The model under review builds one solid part; all positions refer to its coordinate system, in mm. Face numbers are marked on the shaded views. A direction names the side the tool comes from. Round coordinates to 2 decimals unless told otherwise and drop trailing zeros. Loops run counter-clockwise (first coordinate to the right, second up) from the corner with the lowest first, then second, coordinate; pieces in that order, holes last. Notation, with made-up numbers: M 34.25,-39.75 L 90.25,-39.75 A35 ccw 90.25,-1.75 Z; hole C 54,-19 d5. An arc over 180 degrees is marked long. Return JSON: item names as keys, results as strings. Group by question number.
Q1. Consider section B-B (z = 17). State the section outline as (x, y) points.
Q2. Clearance check with flat-ended pins moving along their axes: pin 1 Ø12.5 at (x, y) = (32, -1.5) entering from -Z; pin 2 Ø2 at (y, z) = (-8.5, 25.5) entering from +X; pin 3 Ø1.5 at (x, z) = (-12.5, 25) entering from +Y; pin 4 Ø2 at (x, z) = (13.5, 22.5) entering from -Y. State where each tip first meets the part, or that it passes through.
Q3. Consider section A-A (y = 24). State the section outline as (x, z) points, and give its area (3 significant figures).
Q4. Consider section D-D (y = -18). State the section outline as (x, z) points.
Q5. Consider section C-C (x = 38.5). State the section outline as (y, z) points.
Q6. To check wall thickness, follow line 1 along X through (y, z) = (17, 23.5); line 2 along Z through (x, y) = (73, 24); line 3 along Z through (x, y) = (-33.5, 21.5). State the ranges of each line that lie inside material, in increasing order.
Q7. For the marked faces 1 and 2, list the 3-axis set-ups (+Z, -Z, +X, -X, +Y, -Y) from which the entire face can be reached by the end or side of a thin tool; tool diameter is ignored.
from build123d import *

# Parameters (mm, degrees)
F1_DEPTH = 72
F3_DEPTH = 2
F4_W     = 23
F4_H     = 4
F5_DEPTH = 25


# Not quite as in the source:
# - a pattern or mirror of a feature is missing from the dataset's text; its kind, count and spacing are read off the source's solid


with BuildPart() as f1:
    # F0 (on Right) → F1 (new body, symmetric)
    with BuildSketch(Plane.YZ):
        Polygon((-22, 23), (-20, 23), (-20, 25), (20, 25), (20, 21), (22, 21), (22, 27), (-22, 27), align=None)
    extrude(amount=F1_DEPTH, both=True)

    # F2 (on face) → F3 (join)
    with BuildSketch(Plane.YZ.offset(72)):
        with BuildLine():
            Line((30, 27), (22, 27))
            Line((22, 27), (8, 27))
            ThreePointArc((8, 27), (12.2327735284, 20.5611792354), (13.7171431429, 13))
            Line((13.7171431429, 13), (22, 13))
            Line((22, 13), (22, 14.7639320225))
            ThreePointArc((22, 14.7639320225), (24, 20), (26, 14.7639320225))
            Line((26, 14.7639320225), (26, 13))
            Line((26, 13), (30, 13))
            Line((30, 13), (30, 27))
        make_face()
    f3 = extrude(amount=F3_DEPTH)

    # F3_copies: F3 across plane
    add(f3.mirror(Plane(origin=(0, 0, 0), x_dir=(0, 0, -1), z_dir=(-1, 0, 0))))

    # F4 (on face) → F5 (cut)
    with BuildSketch(Plane(origin=(0, 22, 0), x_dir=(-1, 0, 0), z_dir=(0, 1, 0))):
        with Locations((46.5, 23)):
            Rectangle(F4_W, F4_H)
    extrude(amount=-F5_DEPTH, mode=Mode.SUBTRACT)


solid = f1.part
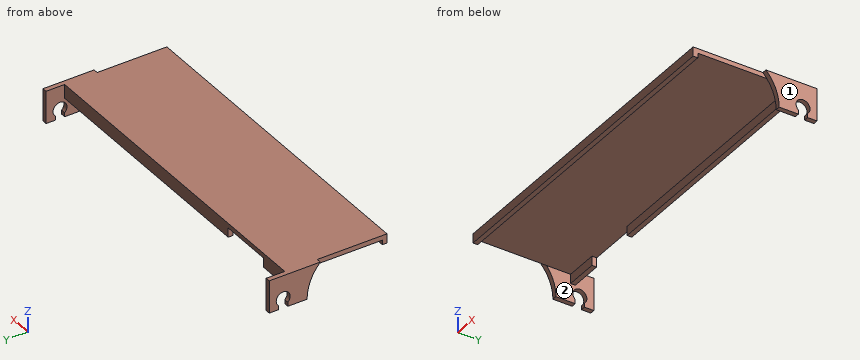
Values:
{
 "1": {"outline": "M -74,13.31 L -72,13.31 L -72,21 L -74,21 Z; M -74,27 L -72,27 L -72,30 L -74,30 Z; M 72,13.31 L 74,13.31 L 74,21 L 72,21 Z; M 72,27 L 74,27 L 74,30 L 72,30 Z"},
 "2": {"pin 1": "stops at z = 25", "pin 2": "stops at x = 72", "pin 3": "stops at y = 22", "pin 4": "stops at y = -22"},
 "3": {"outline": "M -74,20 L -72,20 L -72,27 L -74,27 Z; M 72,20 L 74,20 L 74,27 L 72,27 Z", "area": "28.0 mm2"},
 "4": {"outline": "M -72,25 L 72,25 L 72,27 L -72,27 Z"},
 "5": {"outline": "M -22,23 L -20,23 L -20,25 L 20,25 L 20,21 L 22,21 L 22,27 L -22,27 Z"},
 "6": {"line 1": "x = -74 to -72, 72 to 74", "line 2": "z = 20 to 27", "line 3": "z = 21 to 27"},
 "7": {"face 1": "+Z, -Z, +X, +Y, -Y", "face 2": "-Z"}
}
